Source: three-view drawing plus pictorial views. Frame: mm from the lowest corner of the part. A direction names the side the tool comes from. Give positions to 0.01 mm unless a question says otherwise; leave off trailing zeros. Write each loop counter-clockwise with the first axis right and the second up, starting at its lowest first coordinate (ties: lowest second). Pieces come first, ordered by that corner, then holes. Notation, with made-up numbers: M -40,-16.75 L 12,-16.75 A18 ccw 12,11.25 Z; hole C 73,89 d1. An arc over 180 degrees is marked long. Return JSON: item names as keys, results as strings.
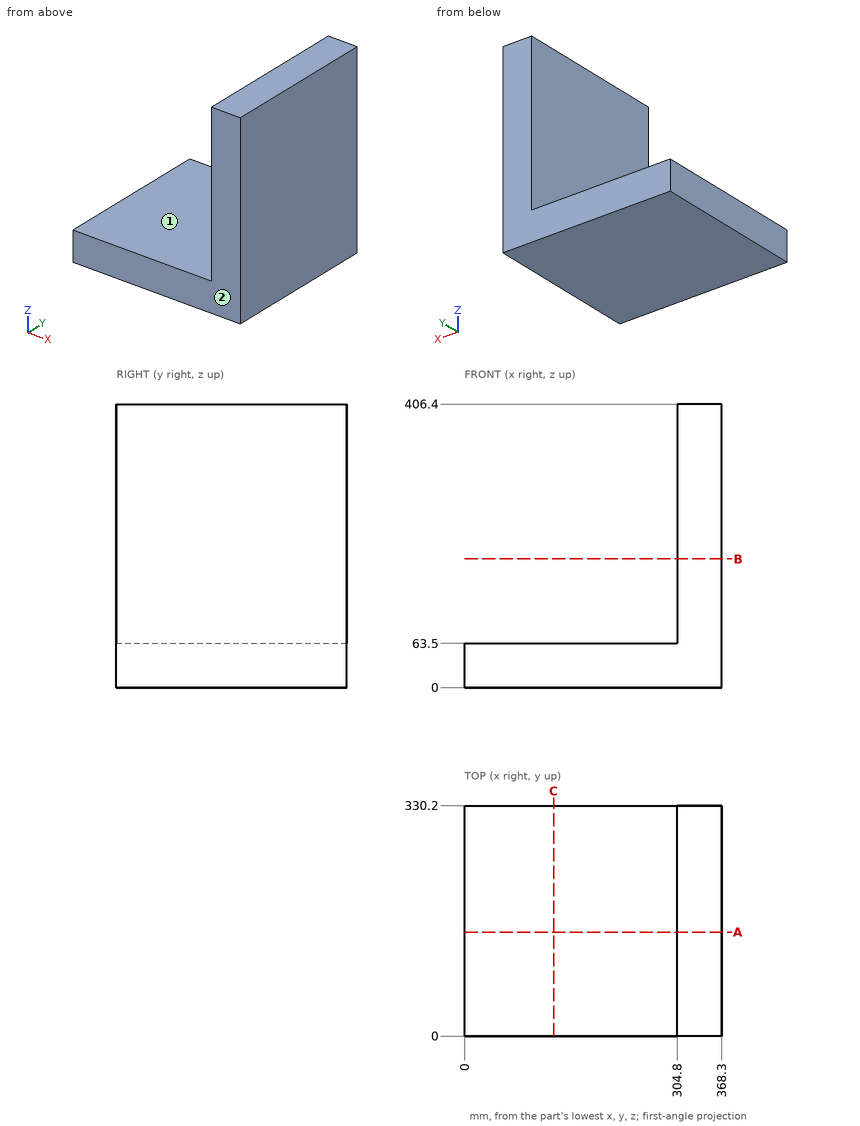
1) Cut plane A-A, the plane y = 149. Return the cut outline in (x, z), then the cut area to 3 significant figures.
Numbers:
{"outline": "M 0,0 L 368.3,0 L 368.3,406.4 L 304.8,406.4 L 304.8,63.5 L 0,63.5 Z", "area": "45,200 mm²"}
2) Contact query for flat-ended pins moving along their axis: pin 1 Ø8 at (x, y) = (223, 40) entering from +Z; pin 2 Ø4 at (y, z) = (177, 351.5) entering from -X; pin 3 Ø2 at (x, y) = (312, 291) entering from -Z. Output: stop coordinate, or through.
Numbers:
{"pin 1": "stops at z = 63.5", "pin 2": "stops at x = 304.8", "pin 3": "stops at z = 0"}
3) Cut plane C-C, the plane x = 127.5. Return the cut outline in (y, z), then the cut area to 3 significant figures.
Numbers:
{"outline": "M 0,0 L 330.2,0 L 330.2,63.5 L 0,63.5 Z", "area": "21,000 mm²"}
4) Cut plane B-B, the plane z = 184.5. Return the cut outline in (x, y), then the cut area to 3 significant figures.
Numbers:
{"outline": "M 304.8,0 L 368.3,0 L 368.3,330.2 L 304.8,330.2 Z", "area": "21,000 mm²"}
5) Line query: line 1 (X direction, y = 239, z = 76.5); line 2 (Z direction, x = 120.5, y = 147.5). Output: solid intervals per line, ascending. Write a range as [from, to].
Numbers:
{"line 1": "x = [304.8, 368.3]", "line 2": "z = [0, 63.5]"}
6) Set-up query: the marked faces 1 and 2. Return all of +Z, -Z, +X, -X, +Y, -Y with unobstructed straight access to the full face (end or side cutting, diameter ignored); none if empty.
Numbers:
{"face 1": "+Z, -X, +Y, -Y", "face 2": "+Z, -Z, +X, -X, -Y"}
